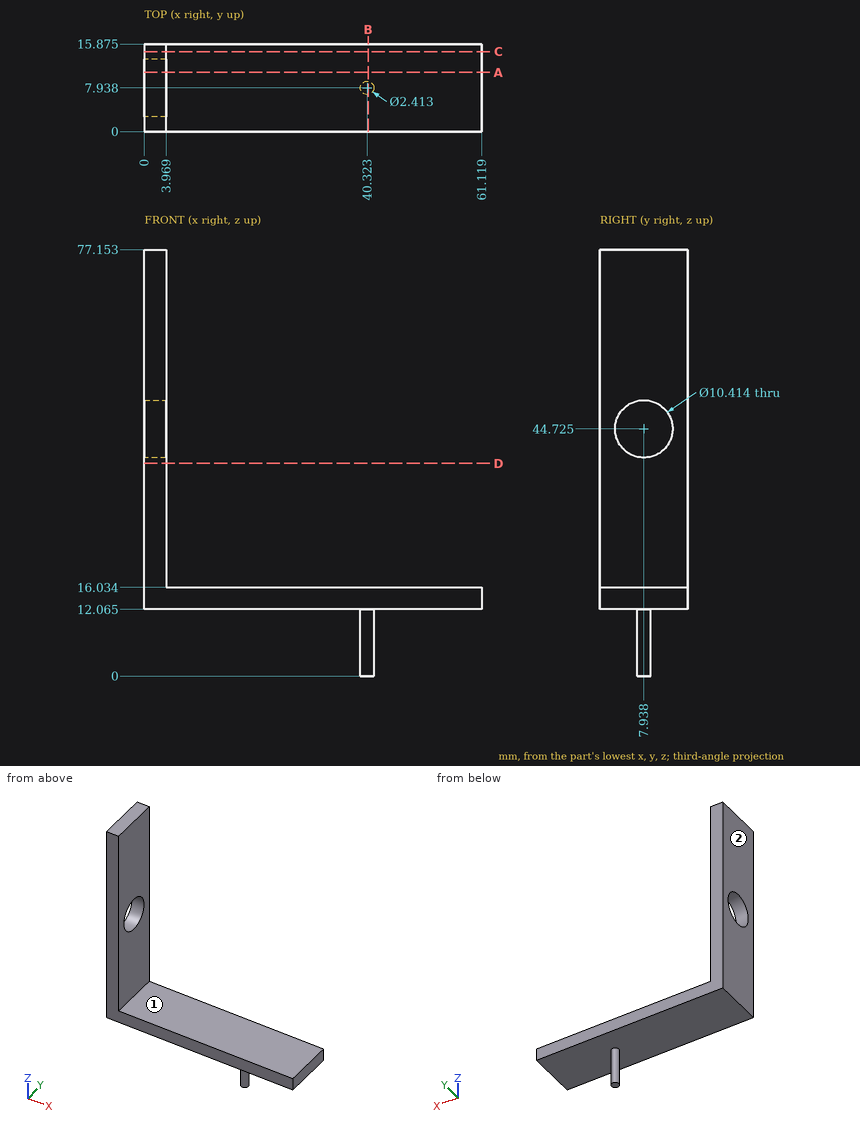
For this review, use the dimensioned drawing (mm, ordinates from the lowest corner) and the shaded views. A direction names the side the tool comes from. Coordinates: 2 decimals unless noted, no trailing zeros. Loops run counter-clockwise (first coordinate to the right, second up) from the corner with the lowest first, then second, coordinate; pieces in that order, holes last. Notation, with made-up numbers: (9, -31.5) - (14, -31.5) arc R26 ccw to (14, 2.5) - close; hole circle Ø3 at (60.25, 60.25). An arc over 180 degrees is marked (long way). Use one line per item in the form item = value. Start each with the question number.
1) Take a section at A-A (y = 10.75). State the section outline as (x, z) points (1 decimal).
2) To check wall thickness, follow probe 1 along Z at (x, y) = (40, 9.75) (1 decimal); probe 2 along X at (y, z) = (6.25, 38.5); probe 3 along Y at (x, z) = (40.5, 6.5) (1 decimal). State the ranges of each line that lie inside material, in increasing order. Write a range as from..to.
3) Take a section at C-C (y = 14.5). State the section outline as (x, z) points (1 decimal).
4) Take a section at B-B (x = 40.5). State the section outline as (y, z) points (1 decimal).
5) For pin 1 (1 mm diameter, centred on x = 29, y = 5, fed in from +Z); pin 2 (3 mm diameter, centred on x = 46, y = 13.5, fed in from -Z) (1 decimal), all flat-tipped, find the tip position at first contact; note any pin that passes through.
6) For the marked faces 1 and 2, list the 3-axis set-ups (+Z, -Z, +X, -X, +Y, -Y) from which the entire face can be reached by the end or side of a thin tool; tool diameter is ignored.
7) Take a section at D-D (z = 38.5). State the section outline as (x, y) points (1 decimal).
From the geometry:
q1.outline = (0, 12.1) - (61.1, 12.1) - (61.1, 16) - (4, 16) - (4, 40.3) - (0, 40.3) - close; (0, 49.1) - (4, 49.1) - (4, 77.2) - (0, 77.2) - close
q2.probe_1 = 12.1..16
q2.probe_2 = 0..3.97
q2.probe_3 = 6.7..9.1
q3.outline = (0, 12.1) - (61.1, 12.1) - (61.1, 16) - (4, 16) - (4, 77.2) - (0, 77.2) - close
q4.outline = (0, 12.1) - (6.7, 12.1) - (6.7, 0) - (9.1, 0) - (9.1, 12.1) - (15.9, 12.1) - (15.9, 16) - (0, 16) - close
q5.pin_1 = 16.03
q5.pin_2 = 12.1
q6.face_1 = +Z, +X, +Y, -Y
q6.face_2 = +Z, -Z, -X, +Y, -Y
q7.outline = (0, 0) - (4, 0) - (4, 15.9) - (0, 15.9) - close
